from build123d import *

# Parameters (mm, degrees)
F0_R     = 1.5
F0_R_2   = 1
F1_DEPTH = 0.3


with BuildPart() as f1:
    # F0 (on Front) → F1 (new body)
    with BuildSketch(Plane.XZ):
        with BuildLine():
            Line((-4, -3), (4, -3))
            Line((4, -3), (4, 3))
            Line((4, 3), (0.85, 3))
            Line((0.85, 3), (0.85, 12.8))
            ThreePointArc((0.85, 12.8), (0, 17.651064), (-0.85, 12.8))
            Line((-0.85, 12.8), (-0.85, 3))
            Line((-0.85, 3), (-4, 3))
            Line((-4, 3), (-4, -3))
        make_face()
        Circle(F0_R, mode=Mode.SUBTRACT)
        with Locations((0, 15.151064)):
            Circle(F0_R_2, mode=Mode.SUBTRACT)
    extrude(amount=F1_DEPTH)


solid = f1.part
CAD build for the part. Positions are in the model's coordinates, mm. Round coordinates to 2 decimals unless told otherwise and drop trailing zeros. Write each loop counter-clockwise with the first axis right and the second up, starting at its lowest first coordinate (ties: lowest second). Pieces come first, ordered by that corner, then holes.
(1) Slice it at A-A, the plane x = 0. Write the cut outline in (y, z), and give its area (3 significant figures).
(2) Slice it at D-D, the plane y = -0.25. Write the cut outline in (x, z), and give its area (3 significant figures).
(3) Probe line 1 along Z through (x, y) = (0, -0.1); line 2 along X through (y, z) = (-0.1, 15.75); line 3 along Z through (x, y) = (-2.25, -0.05). List the from-to ranges inside material, lowest first.
(4) Slice it at B-B, the plane z = 0. Write the cut outline in (x, y), and give its area (3 significant figures).
(5) Mould opens along Z. For faces 1 (the face through (0, 0, 5)), 2 (the face through (0.1, -0.15, 17.65)), 3 (the face through (-1.19, -0.15, -0.91)) say: pulls with the +Z half, pulls with the -Z half, needs draft (parallel to the pull), parting line crosses it, or undercut.
(6) Slice it at C-C, the plane x = -2.25. Write the cut outline in (y, z), and give its area (3 significant figures).
From the geometry:
1. outline: (-0.3, -3) - (0, -3) - (0, -1.5) - (-0.3, -1.5) - close; (-0.3, 1.5) - (0, 1.5) - (0, 14.15) - (-0.3, 14.15) - close; (-0.3, 16.15) - (0, 16.15) - (0, 17.65) - (-0.3, 17.65) - close
1. area: 4.70 mm2
2. outline: (-4, -3) - (4, -3) - (4, 3) - (0.85, 3) - (0.85, 12.8) arc R2.5 ccw (long way) to (-0.85, 12.8) - (-0.85, 3) - (-4, 3) - close; hole circle Ø3 at (0, 0); hole circle Ø2 at (0, 15.15)
2. area: 73.9 mm2
3. line 1: z = -3 to -1.5, 1.5 to 14.15, 16.15 to 17.65
3. line 2: x = -2.43 to -0.8, 0.8 to 2.43
3. line 3: z = -3 to 3, 14.06 to 16.24
4. outline: (-4, -0.3) - (-1.5, -0.3) - (-1.5, 0) - (-4, 0) - close; (1.5, -0.3) - (4, -0.3) - (4, 0) - (1.5, 0) - close
4. area: 1.50 mm2
5. face 1: needs draft
5. face 2: undercut
5. face 3: undercut
6. outline: (-0.3, -3) - (0, -3) - (0, 3) - (-0.3, 3) - close; (-0.3, 14.06) - (0, 14.06) - (0, 16.24) - (-0.3, 16.24) - close
6. area: 2.45 mm2
